Build history of the part. All positions in model axes, mm. A direction names the side the tool comes from. Coordinates: 2 decimals unless noted, no trailing zeros. Loops run counter-clockwise (first coordinate to the right, second up) from the corner with the lowest first, then second, coordinate; pieces in that order, holes last.
Item 1: Drill centre lines: line 1 along X through (y, z) = (-107.5, -2.8); line 2 along Y through (x, z) = (-27, -2); line 3 along X through (y, z) = (-100, 11). Where is each one in solid material? Low to high.
Item 2: Cut at B-B (x = -22). List the corners of the cut face in (y, z), and give its area (3 significant figures).
Item 3: Cut at C-C (z = 11.5). List the corners of the cut face in (x, y), and give its area (3 significant figures).
Item 4: 3-axis set-ups, long thin cutter, end or side, ignore diameter. For faces 1 (the face through (-10, 125, -1)), 2 (the face through (0, -43, 23)): which of +Z, -Z, +X, -X, +Y, -Y reach the whole face in a straight line?
Item 5: Flat gauge pins, fed straight in: pin 1 (6.5 mm diameter, centred on y = 107.5, z = 27.25, fed in from -X); pin 2 (4.5 mm diameter, centred on x = -37.25, y = 107.5, fed in from +Z). Where does each tip first touch, or does it go through?
Item 6: Cut at A-A (y = -57). List the corners of the cut face in (x, z).
from build123d import *

# Parameters (mm, degrees)
F0_W           = 4
F0_H           = 46
F1_DEPTH       = 125
F4_D           = 4
F4_DEPTH       = 15
F4_TIP         = 1.2017212381
F4_ON_F2_D     = 4
F4_ON_F2_DEPTH = 15
F4_ON_F2_TIP   = 1.2017212381
F6_DEPTH       = 90


with BuildPart() as f1:
    # F0 (on Front) → F1 (new body)
    with BuildSketch(Plane.XZ):
        with Locations((2, 23)):
            Rectangle(F0_W, F0_H)
        Polygon((4, 0), (0, 0), (-46, 0), (-46, -4), (4, -4), align=None)
    extrude(amount=F1_DEPTH)

    # F4
    with Locations(Plane.YZ.offset(4)):
        with Locations((-117.5, 37.25), (-107.5, 37.25), (-107.5, 27.25), (-117.5, 27.25)):
            Hole(F4_D / 2, depth=F4_DEPTH)
            with Locations((0, 0, -(F4_DEPTH + F4_TIP / 2))):  # 118° drill point
                Cone(0, F4_D / 2, F4_TIP, mode=Mode.SUBTRACT)

    # F4 on F2
    with Locations(Plane(origin=(0, 0, -4), x_dir=(1, 0, 0), z_dir=(0, 0, -1))):
        with Locations((-27.25, 117.5), (-37.25, 117.5), (-37.25, 107.5), (-27.25, 107.5)):
            Hole(F4_ON_F2_D / 2, depth=F4_ON_F2_DEPTH)
            with Locations((0, 0, -(F4_ON_F2_DEPTH + F4_ON_F2_TIP / 2))):  # 118° drill point
                Cone(0, F4_ON_F2_D / 2, F4_ON_F2_TIP, mode=Mode.SUBTRACT)

    # F5: F1 across face


with BuildPart() as f1_1:
    add(f1.part)
    add(f1.part.mirror(Plane(origin=(-9.9791666667, 0, 9.9791666667), x_dir=(1, 0, 0), z_dir=(0, 1, 0))))

    # F6 (add): a face of the model
    f6_faces = [f1_1.faces().sort_by_distance(p)[0] for p in [
        (0.7071067812, -125, 23),
    ]]
    extrude(f6_faces, amount=F6_DEPTH)


solid = f1_1.part
Filled sheet:
1. line 1: x = -46 to -39.25, -35.25 to -29.25, -25.25 to 4
1. line 2: y = -215 to -119.48, -115.52 to -109.48, -105.52 to 105.52, 109.48 to 115.52, 119.48 to 125
1. line 3: x = 0 to 4
2. outline: (-215, -4) - (125, -4) - (125, 0) - (-215, 0) - close
2. area: 1,360 mm2
3. outline: (0, -215) - (4, -215) - (4, 125) - (0, 125) - close
3. area: 1,360 mm2
4. face 1: +Z, -Z, +X, -X, +Y
4. face 2: +Z, -X, +Y, -Y
5. pin 1: stops at x = 0
5. pin 2: stops at z = 0
6. outline: (-46, -4) - (4, -4) - (4, 46) - (0, 46) - (0, 0) - (-46, 0) - close
